```python
from build123d import *

# Parameters (mm, degrees)
SKETCH1_R           = 0.75
BOSS_EXTRUDE1_DEPTH = 1
SKETCH3_R           = 3.75
BOSS_EXTRUDE2_DEPTH = 5
SKETCH3_3_R         = 1.5
CUT_EXTRUDE1_DEPTH  = 19.347343132
SKETCH1_2_R         = 0.75
CUT_EXTRUDE2_DEPTH  = 19.347343132
SKETCH4_R           = 2.355
CUT_EXTRUDE3_DEPTH  = 2
CUT_EXTRUDE4_DEPTH  = 2
CIRPATTERN1_COUNT   = 56


with BuildPart() as part:
    # Sketch1 → Boss-Extrude1 (new body)
    with BuildSketch(Plane(origin=(0, 0, 0), x_dir=(1, 0, 0), z_dir=(0, 1, 0))):
        with BuildLine():
            Line((-2.49119588, 14.959626071), (-3.75, 0))
            Line((-3.75, 0), (-2.49119588, -14.959626071))
            ThreePointArc((-2.49119588, -14.959626071), (0, -17.25), (2.49119588, -14.959626071))
            Line((2.49119588, -14.959626071), (3.75, 0))
            Line((3.75, 0), (2.49119588, 14.959626071))
            ThreePointArc((2.49119588, 14.959626071), (0, 17.25), (-2.49119588, 14.959626071))
        make_face()
        with Locations(Location((0, 14.75, 0), (0, 0, 270))):
            Circle(SKETCH1_R, mode=Mode.SUBTRACT)
        with Locations(Location((0, 12.75, 0), (0, 0, 270))):
            Circle(SKETCH1_R, mode=Mode.SUBTRACT)
        with Locations(Location((0, 10.75, 0), (0, 0, 270))):
            Circle(SKETCH1_R, mode=Mode.SUBTRACT)
        with Locations(Location((0, 8.75, 0), (0, 0, 270))):
            Circle(SKETCH1_R, mode=Mode.SUBTRACT)
        with Locations(Location((0, 6.75, 0), (0, 0, 270))):
            Circle(SKETCH1_R, mode=Mode.SUBTRACT)
        with Locations(Location((0, 4.75, 0), (0, 0, 270))):
            Circle(SKETCH1_R, mode=Mode.SUBTRACT)
        with Locations(Location((0, 0, 0), (0, 0, 270))):
            Circle(SKETCH1_R, mode=Mode.SUBTRACT)
        with Locations(Location((0, -14.75, 0), (0, 0, 90))):
            Circle(SKETCH1_R, mode=Mode.SUBTRACT)
        with Locations(Location((0, -12.75, 0), (0, 0, 90))):
            Circle(SKETCH1_R, mode=Mode.SUBTRACT)
        with Locations(Location((0, -10.75, 0), (0, 0, 90))):
            Circle(SKETCH1_R, mode=Mode.SUBTRACT)
        with Locations(Location((0, -8.75, 0), (0, 0, 90))):
            Circle(SKETCH1_R, mode=Mode.SUBTRACT)
        with Locations(Location((0, -6.75, 0), (0, 0, 90))):
            Circle(SKETCH1_R, mode=Mode.SUBTRACT)
        with Locations(Location((0, -4.75, 0), (0, 0, 90))):
            Circle(SKETCH1_R, mode=Mode.SUBTRACT)
    extrude(amount=BOSS_EXTRUDE1_DEPTH)

    # Sketch3 → Boss-Extrude2 (add)
    with BuildSketch(Plane.XZ):
        with Locations(Location((0, 0, 0), (0, 0, 9.619846544))):
            Circle(SKETCH3_R)
    extrude(amount=BOSS_EXTRUDE2_DEPTH)

    # Sketch3<3> → Cut-Extrude1 (cut, through all)
    with BuildSketch(Plane.XZ):
        with Locations(Location((0, 0, 0), (0, 0, 270))):
            Circle(SKETCH3_3_R)
    extrude(amount=-CUT_EXTRUDE1_DEPTH, mode=Mode.SUBTRACT)

    # Sketch1<2> → Cut-Extrude2 (cut, through all)
    with BuildSketch(Plane(origin=(0, 0, 0), x_dir=(1, 0, 0), z_dir=(0, 1, 0))):
        with Locations(Location((0, 0, 0), (0, 0, 270))):
            Circle(SKETCH1_2_R)
    extrude(amount=-CUT_EXTRUDE2_DEPTH, mode=Mode.SUBTRACT)

    # Sketch4 → Cut-Extrude3 (cut)
    with BuildSketch(Plane.XZ.offset(5)):
        with Locations(Location((0, 0, 0), (0, 0, 270))):
            Circle(SKETCH4_R)
    extrude(amount=-CUT_EXTRUDE3_DEPTH, mode=Mode.SUBTRACT)

    # Sketch5 → Cut-Extrude4 (cut)
    with BuildSketch(Plane.XZ.offset(5)):
        with BuildLine():
            Line((-0.141421356, 2.35074988), (0, 2.492171237))
            Line((0, 2.492171237), (0.141421356, 2.35074988))
            ThreePointArc((0.141421356, 2.35074988), (0, 2.355), (-0.141421356, 2.35074988))
        make_face()
    cut_extrude4 = extrude(amount=-CUT_EXTRUDE4_DEPTH, mode=Mode.SUBTRACT)

    # CirPattern1: Cut-Extrude4 ×56 about axis
    cirpattern1_axis = Axis((0, 0, 0), (0, 1, 0))
    for i in range(1, CIRPATTERN1_COUNT):
        add(cut_extrude4.rotate(cirpattern1_axis, i * 360 / CIRPATTERN1_COUNT), mode=Mode.SUBTRACT)


solid = part.part
```
Here's how the part is built. I have some questions about the finished solid (model axes, mm). A direction names the side the tool comes from. Round coordinates to 2 decimals unless told otherwise and drop trailing zeros. Order: outer loops, then holes, each group sorted by start corner. A loop starts at its lowest first (then second) coordinate and runs counter-clockwise, first axis right, second up. Notation, with made-up numbers: M 58.25,-14.5 L 85.25,-14.5 A9 ccw 85.25,-0.5 Z; hole C 81.25,84 d3. An arc over 180 degrees is marked long. Answer as CSV lines item,"result".
Item 1: We'd pull the mould along Z, two halves only. Please class faces 1 (the cylindrical face through (0.05, 0.49, -17.25)), 2 (the cylindrical face through (0, 0.5, 13.5)), 3 (the flat face through (1, 0, -9)): +Z half, -Z half, draft (parallel to the pull), parting line (faces both ways), or undercut.
From the geometry:
face 1,"-Z half"
face 2,"undercut"
face 3,"draft"
Item 2: Imagine slicing it at B-B on y = -2.2. List the corners of the cut face in (x, z) for me.
From the geometry:
outline,"C 0,0 d7.5; hole C 0,0 d1.5"
Item 3: Imagine slicing it at D-D on z = 10.75. List the corners of the cut face in (x, y) for me.
From the geometry:
outline,"M -2.85,0 L -0.75,0 L -0.75,1 L -2.85,1 Z; M 0.75,0 L 2.85,0 L 2.85,1 L 0.75,1 Z"
Item 4: Imagine slicing it at A-A on z = -8.5. List the corners of the cut face in (x, y) for me.
From the geometry:
outline,"M -3.03,0 L -0.71,0 L -0.71,1 L -3.03,1 Z; M 0.71,0 L 3.03,0 L 3.03,1 L 0.71,1 Z"
Item 5: Please list where these lines run through material, in increasing order: L1, parallel to X at y = 0.45, z = 0; L2, parallel to Y at x = -0.75, z = 11; L3, parallel to X at y = 0.55, z = 8.75. Write a range as [from, to].
From the geometry:
L1,"[-3.75, -1.5], [1.5, 3.75]"
L2,"[0, 1]"
L3,"[-3.01, -0.75], [0.75, 3.01]"
Item 6: Imagine slicing it at C-C on x = 3. List the corners of the cut face in (y, z) for me, and give its area (3 significant figures).
From the geometry:
outline,"M -5,-2.25 L 0,-2.25 L 0,-8.91 L 1,-8.91 L 1,8.91 L 0,8.91 L 0,2.25 L -5,2.25 Z"
area,"40.3 mm2"
Item 7: Which directions (+Z, -Z, +X, -X, +Y, -Y) give clear straight access to the entire face, cutting with the end or side of a thin tool? Please do faces 4 (the flat face through (3, -5, 0)), 5 (the cylindrical face through (3.338, -2.465, 1.708)).
From the geometry:
face 4,"+Z, -Z, +X, -X, -Y"
face 5,"-Y"
Item 8: For pin 1 (0.9 mm diameter, centred on x = 0, z = -4.75, fed in from -Y); pin 2 (2 mm diameter, centred on y = 0, z = 5.5, fed in from +X); pin 3 (0.9 mm diameter, centred on x = -0.5, z = 0.5, fed in from +Y); pin 4 (3.5 mm diameter, centred on x = 0, z = -6, fed in from -Y), each with a flat end and sliding along its axis, tell me the tip position at first contact or that it passes through.
From the geometry:
pin 1,"through"
pin 2,"x = 3.37"
pin 3,"y = 0"
pin 4,"y = 0"
